Check sheet for the modelled part. Datum: model origin and axes. Units: mm. A direction names the side the tool comes from. Give positions to 0.01 mm unless a question says otherwise; leave off trailing zeros. Loops run counter-clockwise (first coordinate to the right, second up) from the corner with the lowest first, then second, coordinate; pieces in that order, holes last.
```python
from build123d import *

# Parameters (mm, degrees)
F0_W     = 203.2
F0_H     = 114.3
F0_R     = 12.7
F1_DEPTH = 20.32
F2_DEPTH = 52.07


with BuildPart() as f1:
    # F0 (on Front) → F1 (new body)
    with BuildSketch(Plane.XZ):
        Rectangle(F0_W, F0_H)
        Polygon((-6.35, -21.997045), (6.35, 0), (19.05, -21.997045), align=None, mode=Mode.SUBTRACT)
        with Locations((-82.55, 0)):
            Circle(F0_R, mode=Mode.SUBTRACT)
        Polygon((-22.225, 9.525), (-22.225, 0), (-22.225, -9.525), (-41.275, -9.525), (-41.275, 0), (-41.275, 9.525), align=None, mode=Mode.SUBTRACT)
    extrude(amount=F1_DEPTH)

    # F0 (on Front) → F2 (join)
    with BuildSketch(Plane.XZ):
        with Locations((-82.55, 0)):
            Circle(F0_R)
        Polygon((-31.75, 0), (-22.225, 0), (-22.225, 9.525), (-41.275, 9.525), (-41.275, 0), align=None)
        Polygon((-22.225, -9.525), (-22.225, 0), (-31.75, 0), (-41.275, 0), (-41.275, -9.525), align=None)
    extrude(amount=F2_DEPTH)


solid = f1.part
```
(1) Material ranges on line 1 (Y direction, x = 62, z = 8.5); line 2 (X direction, y = -30.5, z = -3.5) (3 decimals); line 3 (Z direction, x = -34, y = -43) (3 decimals), recorded low to high.
(2) Section check B-B on x = -82.55. Record the boundary of the cut face in (y, z), plus the area to 3 significant figures.
(3) Section check A-A on y = -22.5. Record the boundary of the cut face in (x, z) (3 decimals), plus the area to 3 significant figures.
(4) Gauge pin test, flat ends, axial feed: pin 1 Ø2 at (x, y) = (-79.5, -38.5) entering from -Z; pin 2 Ø3 at (x, z) = (40.5, 24.5) entering from -Y; pin 3 Ø21 at (y, z) = (-38, -0.5) entering from +X (3 decimals). Record the tip position at first contact, or that the pin passes through.
(5) Release check for a two-part mould opening along Z. For faces 4 (the face through (-32, -36, 9.525)), 5 (the face through (-1, 0, 1)), 6 (the face through (7, -10, -21.997)) record: pulls with the +Z half, pulls with the -Z half, needs draft (parallel to the pull), parting line crosses it, or undercut.
(6) Access from +Z, -Z, +X, -X, +Y, -Y to the whole of each face (thin tool, end or side, straight path). Record for faces 1 (the face through (-22.225, -36, 0)), 2 (the face through (0, -10, -11)), 3 (the face through (-41.275, -36, 0)).
(7) Section check C-C on x = -2. Record the boundary of the cut face in (y, z).
(8) Section check D-D on z = 26.5. Record the boundary of the cut face in (x, y).
Computed values:
1. line 1: y = -20.32 to 0
1. line 2: x = -94.758 to -70.342, -41.275 to -22.225
1. line 3: z = -9.525 to 9.525
2. outline: (-52.07, -12.7) - (-20.32, -12.7) - (-20.32, -57.15) - (0, -57.15) - (0, 57.15) - (-20.32, 57.15) - (-20.32, 12.7) - (-52.07, 12.7) - close
2. area: 3,130 mm2
3. outline: circle Ø25.4 at (-82.55, 0); (-41.275, -9.525) - (-22.225, -9.525) - (-22.225, 9.525) - (-41.275, 9.525) - close
3. area: 870 mm2
4. pin 1: stops at z = -12.53
4. pin 2: stops at y = -20.32
4. pin 3: stops at x = -22.225
5. face 4: pulls with the +Z half
5. face 5: needs draft
5. face 6: undercut
6. face 1: +Z, -Z, +X, -Y
6. face 2: +Y, -Y
6. face 3: +Z, -Z, -Y
7. outline: (-20.32, -57.15) - (0, -57.15) - (0, -22) - (-20.32, -22) - close; (-20.32, -14.46) - (0, -14.46) - (0, 57.15) - (-20.32, 57.15) - close
8. outline: (-101.6, -20.32) - (101.6, -20.32) - (101.6, 0) - (-101.6, 0) - close
